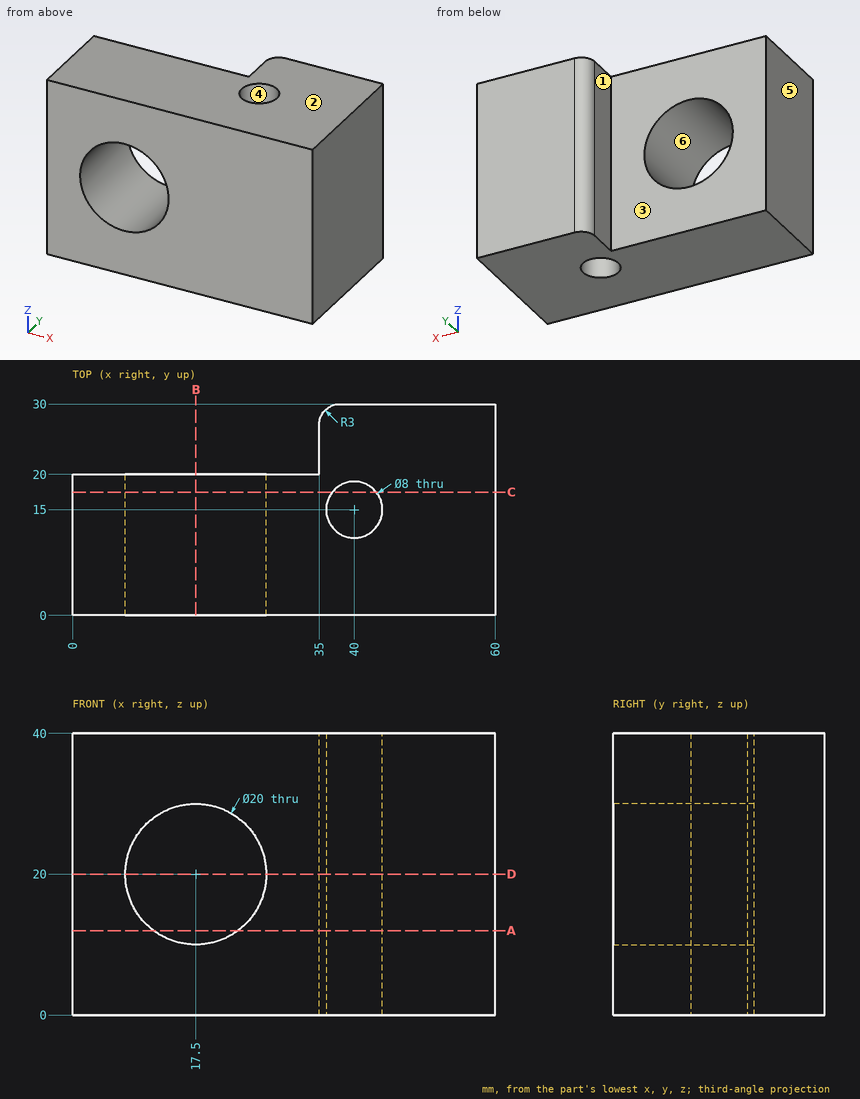
Verification items for this drawing (mm, ordinates from the low corner). A direction names the side the tool comes from. Round coordinates to 2 decimals unless told otherwise and drop trailing zeros. Write each loop counter-clockwise with the first axis right and the second up, starting at its lowest first coordinate (ties: lowest second). Pieces come first, ordered by that corner, then holes. Notation, with made-up numbers: (56, -32) - (71, -32) arc R18 ccw to (71, -8) - close; hole circle Ø8 at (22, 65.25). An arc over 180 degrees is marked (long way). Answer as a JSON object with one key per item and string values. Group by question number.
Q1. Mould release check, pull along X, two halves, no side actions. Record for the marked faces 3, 4, 5 and 6: released by +X, released by -X, zero draft, split by the parting line, or undercut.
Q2. Section check D-D, the plane z = 20. Enter the section's corners in (x, y).
Q3. Section check C-C, the plane y = 17.5. Enter the section's corners in (x, z), plus the area to 3 significant figures.
Q4. Section check B-B, the plane x = 17.5. Enter the section's corners in (y, z).
Q5. Thickness scan on line 1 (Y direction, x = 40, z = 26); line 2 (Z direction, x = 18, y = 16.25); line 3 (X direction, y = 13, z = 13.5). Record the ranges inside material, lowest first.
Q6. Go/stop test with flat-tipped pins: pin 1 Ø10 at (x, z) = (22, 30.5) entering from +Y; pin 2 Ø7 at (x, y) = (40, 15) entering from +Z; pin 3 Ø5.5 at (y, z) = (24, 25.5) entering from -X. Record where each tip stops, or that it passes through.
Q7. Tool access check on the marked faces 1 and 2. Record the directions out of +Z, -Z, +X, -X, +Y, -Y that give a thin tool (end or side, any length) a straight path to the whole face; none if there is none.
Q8. Section check A-A, the plane z = 12. Enter the section's corners in (x, y).
Found:
{
 "1": {"face 3": "zero draft", "face 4": "undercut", "face 5": "released by -X", "face 6": "undercut"},
 "2": {"outline": "(0, 0) - (7.5, 0) - (7.5, 20) - (0, 20) - close; (27.5, 0) - (60, 0) - (60, 30) - (38, 30) arc R3 ccw to (35, 27) - (35, 20) - (27.5, 20) - close; hole circle Ø8 at (40, 15)"},
 "3": {"outline": "(0, 0) - (36.88, 0) - (36.88, 40) - (0, 40) - close; (43.12, 0) - (60, 0) - (60, 40) - (43.12, 40) - close; hole circle Ø20 at (17.5, 20)", "area": "1,840 mm^2"},
 "4": {"outline": "(0, 0) - (20, 0) - (20, 10) - (0, 10) - close; (0, 30) - (20, 30) - (20, 40) - (0, 40) - close"},
 "5": {"line 1": "y = 0 to 11, 19 to 30", "line 2": "z = 0 to 10.01, 29.99 to 40", "line 3": "x = 0 to 9.9, 25.1 to 36.54, 43.46 to 60"},
 "6": {"pin 1": "stops at y = 20", "pin 2": "passes through", "pin 3": "stops at x = 35"},
 "7": {"face 1": "+Z, -Z, -X, +Y", "face 2": "+Z, +X, -X, +Y, -Y"},
 "8": {"outline": "(0, 0) - (11.5, 0) - (11.5, 20) - (0, 20) - close; (23.5, 0) - (60, 0) - (60, 30) - (38, 30) arc R3 ccw to (35, 27) - (35, 20) - (23.5, 20) - close; hole circle Ø8 at (40, 15)"}
}
